Read the model definition and answer for the solid it produces. Units are mm, in the model's axes. A direction names the side the tool comes from. Coordinates: 2 decimals unless noted, no trailing zeros. Loops run counter-clockwise (first coordinate to the right, second up) from the corner with the lowest first, then second, coordinate; pieces in that order, holes last. Notation, with made-up numbers: M 78,-13 L 108,-13 A18 cw 108,18 Z; hole C 25,35 d6. An arc over 180 degrees is marked long. One line per item, written item: value. Start each with the question number.
```python
from build123d import *

# Parameters (mm, degrees)
SKETCH1_W           = 35
SKETCH1_H           = 60
SKETCH1_W_2         = 31
SKETCH1_H_2         = 56
BOSS_EXTRUDE1_DEPTH = 45
SKETCH2_W           = 30
SKETCH2_H           = 12
BOSS_EXTRUDE2_DEPTH = 16.5
SKETCH3_R           = 5
BOSS_EXTRUDE3_DEPTH = 10
SKETCH4_W           = 6.5
SKETCH4_H           = 2
BOSS_EXTRUDE4_DEPTH = 17.5
BOSS_EXTRUDE5_REACH = 73.753
SKETCH5_W           = 5
SKETCH5_H           = 2
BOSS_EXTRUDE6_REACH = 73.502
FILLET1_R           = 2


with BuildPart() as part:
    # Sketch1 → Boss-Extrude1 (new body)
    with BuildSketch(Plane(origin=(0, 0, 0), x_dir=(-1, 0, 0), z_dir=(0, 1, 0))):
        Rectangle(SKETCH1_W, SKETCH1_H)
        Rectangle(SKETCH1_W_2, SKETCH1_H_2, mode=Mode.SUBTRACT)
    extrude(amount=BOSS_EXTRUDE1_DEPTH)

    # Sketch2 → Boss-Extrude2 (add)
    with BuildSketch(Plane(origin=(15.5, 0, 0), x_dir=(0, -1, 0), z_dir=(-1, 0, 0))):
        with Locations((-15, 0)):
            Rectangle(SKETCH2_W, SKETCH2_H)
    extrude(amount=BOSS_EXTRUDE2_DEPTH)

    # Sketch3 → Boss-Extrude3 (add)
    with BuildSketch(Plane(origin=(-1, 0, 0), x_dir=(0, -1, 0), z_dir=(-1, 0, 0))):
        with Locations(Location((-22.5, 0, 0), (0, 0, 270))):
            Circle(SKETCH3_R)
    extrude(amount=BOSS_EXTRUDE3_DEPTH)

    # Sketch4 → Boss-Extrude4 (add)
    with BuildSketch(Plane(origin=(0, 45, 0), x_dir=(-1, 0, 0), z_dir=(0, 1, 0))):
        with Locations((14.25, 29)):
            Rectangle(SKETCH4_W, SKETCH4_H)
        with Locations((-2.25, 29)):
            Rectangle(SKETCH4_W, SKETCH4_H)
    boss_extrude4 = extrude(amount=BOSS_EXTRUDE4_DEPTH)

    # Sketch5 → Boss-Extrude5 (add, up to next)
    with BuildSketch(Plane(origin=(-1, 0, 0), x_dir=(0, -1, 0), z_dir=(-1, 0, 0)), mode=Mode.PRIVATE) as boss_extrude5_sk1:
        with Locations((-60, 29)):
            Rectangle(SKETCH5_W, SKETCH5_H)
    boss_extrude5_tool1 = extrude(boss_extrude5_sk1.sketch, amount=BOSS_EXTRUDE5_REACH, mode=Mode.PRIVATE) - part.part
    boss_extrude5 = boss_extrude5_tool1.solids().sort_by_distance((-1, 60, 29))[0]
    add(boss_extrude5)

    # Mirror1: Boss-Extrude4, Boss-Extrude5 across plane
    add(boss_extrude4.mirror(Plane.XY))
    add(boss_extrude5.mirror(Plane.XY))

    # Boss-Extrude6: up to this face of the body (flat: up to its plane)
    boss_extrude6_end = Plane(part.part.faces().sort_by_distance((2.554270463, 0, 0))[0])
    # Sketch7 → Boss-Extrude6 (add, up to the picked face)
    with BuildSketch(Plane(origin=(0, 62.5, 0), x_dir=(-1, 0, 0), z_dir=(0, 1, 0)), mode=Mode.PRIVATE) as boss_extrude6_sk1:
        with BuildLine():
            Line((11, 30), (17.5, 30))
            Line((17.5, 30), (17.5, 20))
            Line((17.5, 20), (13, 20))
            ThreePointArc((13, 20), (11.585786438, 20.585786438), (11, 22))
            Line((11, 22), (11, 30))
        make_face()
    boss_extrude6_tool1 = split(extrude(boss_extrude6_sk1.sketch, amount=-BOSS_EXTRUDE6_REACH, mode=Mode.PRIVATE), bisect_by=boss_extrude6_end, keep=Keep.BOTH, mode=Mode.PRIVATE)
    # Sketch7 → Boss-Extrude6 (add, up to the picked face)
    with BuildSketch(Plane(origin=(0, 62.5, 0), x_dir=(-1, 0, 0), z_dir=(0, 1, 0)), mode=Mode.PRIVATE) as boss_extrude6_sk2:
        with BuildLine():
            Line((-5.5, 30), (1, 30))
            Line((1, 30), (1, 22))
            ThreePointArc((1, 22), (0.414213562, 20.585786438), (-1, 20))
            Line((-1, 20), (-5.5, 20))
            Line((-5.5, 20), (-5.5, 30))
        make_face()
    boss_extrude6_tool2 = split(extrude(boss_extrude6_sk2.sketch, amount=-BOSS_EXTRUDE6_REACH, mode=Mode.PRIVATE), bisect_by=boss_extrude6_end, keep=Keep.BOTH, mode=Mode.PRIVATE)
    boss_extrude6_1 = boss_extrude6_tool1.solids().sort_by(Axis((-14.287516, 62.5, 25.060936), (0, -1, 0)))[0]
    add(boss_extrude6_1)
    boss_extrude6_2 = boss_extrude6_tool2.solids().sort_by(Axis((2.287516, 62.5, 25.060936), (0, -1, 0)))[0]
    add(boss_extrude6_2)
    boss_extrude6 = boss_extrude6_1 + boss_extrude6_2  # Boss-Extrude6 as one shape, for the pattern or mirror that repeats it

    # Fillet1
    fillet1_edges = [part.edges().sort_by_distance(p)[0] for p in [
        (-15.5, 22.5, 20),
        (-16.5, 45, 20),
        (-11, 22.5, 28),
        (-1, 22.5, 28),
        (5.5, 22.5, 28),
        (5.5, 31.25, 20),
        (15.5, 22.5, 28),
        (5.5, 45, 29),
        (17.5, 22.5, 30),
        (-17.5, 31.25, 30),
    ]]
    fillet(fillet1_edges, radius=FILLET1_R)

    # Mirror2: Boss-Extrude4, Boss-Extrude5, Boss-Extrude6 across plane
    add(boss_extrude4.mirror(Plane.XY))
    add(boss_extrude5.mirror(Plane.XY))
    add(boss_extrude6.mirror(Plane.XY))


solid = part.part
```
1) Section A-A (z = 12) is taken. Determine the outline of the cut face in (x, y).
2) Section D-D (z = 19) is taken. Determine the outline of the cut face in (x, y).
3) For a pull along X with two mould halves and no side action, classify faces 4 (the face through (-11, 22, 0)), 5 (the face through (-5.8, 62.5, 28.3)), 6 (the face through (-11.6, 31.69, -20.57)), 7 (the face through (5.9, 45.8, 28.5)) as released by +X, released by -X, zero draft, split by the parting line, or undercut.
4) Flat-ended cylindrical pins translate along their axes: pin 1 (1 mm diameter, centred on x = -16.5, z = 2, fed in from +Y); pin 2 (9.5 mm diameter, centred on x = 8.5, z = -5.5, fed in from +Y); pin 3 (1.5 mm diameter, centred on x = 13, z = 17.5, fed in from +Y). Find the tip coordinate at first contact, or state that the pin passes through.
5) Consider line 1 along Z through (x, y) = (11.5, 29.5); line 2 along X through (y, z) = (25, -25); line 3 along X through (y, z) = (25, -13). Determine where each line is inside the solid, lowest interval first.
6) A tool of negligible diameter and unlimited length cuts with its end or side. For faces 1 (the face through (-6, 45, -29)), 2 (the face through (-1.6, 22.82, 27.43)), 3 (the face through (-15, 39, -20)), from which of +Z, -Z, +X, -X, +Y, -Y can it reach the whole face along a straight path? Write none if from no direction.
7) Section C-C (z = 0) is taken. Determine the outline of the cut face in (x, y).
Results found:
1. outline: M -17.5,0 L -15.5,0 L -15.5,45 L -17.5,45 Z; M 15.5,0 L 17.5,0 L 17.5,45 L 15.5,45 Z
2. outline: M -17.5,0 L -15.23,0 L -15.23,45.27 L -17.5,45.27 Z; M 15.5,0 L 17.5,0 L 17.5,45 L 15.5,45 Z
3. face 4: undercut
3. face 5: zero draft
3. face 6: undercut
3. face 7: released by +X
4. pin 1: stops at y = 45
4. pin 2: stops at y = 30
4. pin 3: passes through
5. line 1: z = -30 to -28, -6 to 6, 28 to 30
5. line 2: x = -17.5 to -11, -1 to 5.5, 15.5 to 17.5
5. line 3: x = -17.5 to -15.5, 15.5 to 17.5
6. face 1: +Z, -Z
6. face 2: +Y, -Y
6. face 3: +Y
7. outline: M -17.5,0 L -15.5,0 L -15.5,45 L -17.5,45 Z; M -11,17.5 L -1,17.5 L -1,0 L 17.5,0 L 17.5,45 L 15.5,45 L 15.5,30 L -1,30 L -1,27.5 L -11,27.5 Z
